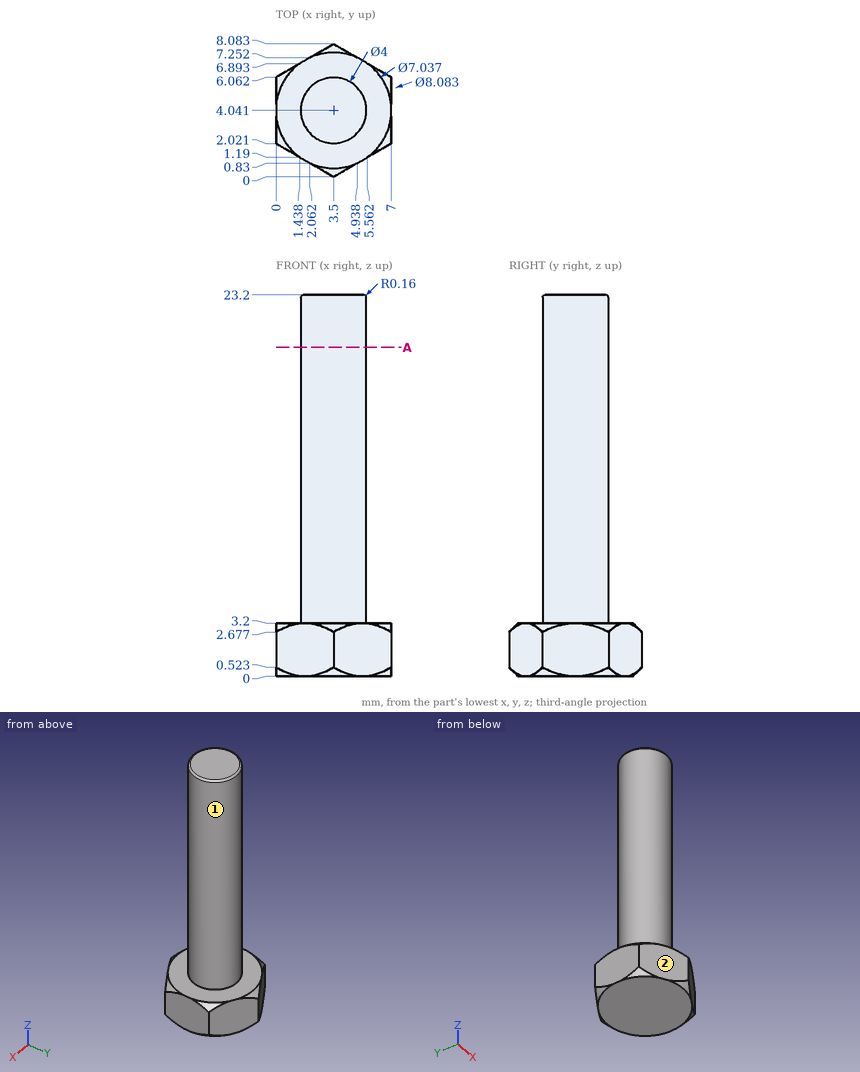
Geometry: see drawing. Coordinates: mm, zero at the bounding-box minimum. A direction names the side the tool comes from. Round coordinates to 2 decimals unless told otherwise and drop trailing zeros. Loops run counter-clockwise (first coordinate to the right, second up) from the corner with the lowest first, then second, coordinate; pieces in that order, holes last. Notation, with made-up numbers: (-20, 71.25) -> (8, 71.25) arc R17 ccw to (8, 83.25) -> close; hole circle Ø1 at (-15, -2). An arc over 180 degrees is marked (long way). One line per question, with ' | ' between items. Start each with the question number.
1. Set-up query: the marked faces 1 and 2. Return all of +Z, -Z, +X, -X, +Y, -Y with unobstructed straight access to the full face (end or side cutting, diameter ignored); none if empty.
2. Section A-A on z = 20. Output: boundary loops of the cut face in (x, y).
3. Line query: line 1 along Z through (x, y) = (3.75, 1.5); line 2 along Y through (x, z) = (3.5, 11.75); line 3 along X through (y, z) = (5.25, 16) (1 decimal). Output: solid intervals per line, ascending. Write a range as [from, to].
4. Contact query for flat-ended pins moving along their axis: pin 1 (3 mm diameter, centred on x = 6.5, z = 13.5, fed in from +Y) (1 decimal); pin 2 (1 mm diameter, centred on x = 3.5, z = 19, fed in from +Y). Output: stop coordinate, or through.
Returned:
1) face 1: +Z | face 2: +Z, -Z, -X, -Y
2) outline: circle Ø4 at (3.5, 4.04)
3) line 1: z = [0, 3.2] | line 2: y = [2.04, 6.04] | line 3: x = [1.9, 5.1]
4) pin 1: stops at y = 5.4 | pin 2: stops at y = 6.04
